from build123d import *

# Parameters (mm, degrees)
F1_R     = 2
F1_W     = 3
F1_H     = 3
F6_DEPTH = 1
F7_DEPTH = 1.6
F5_W     = 3
F5_H     = 3
F8_DEPTH = 1


with BuildPart() as f6:
    # F1 (on Top) → F6 (new body, through all)
    with BuildSketch(Plane.XY):
        with BuildLine():
            ThreePointArc((-30.5, -38), (-27.318019, -36.681981), (-26, -33.5))
            ThreePointArc((-26, -33.5), (-29.882129, -29.04262), (-34.830327, -32.275961))
            ThreePointArc((-34.830327, -32.275961), (-34.088744, -36.214943), (-30.5, -38))
        make_face()
        with Locations((-30.5, -33.5)):
            Circle(F1_R, mode=Mode.SUBTRACT)
        with BuildLine():
            ThreePointArc((-34.830327, -32.275961), (-29.882129, -29.04262), (-26, -33.5))
            ThreePointArc((-26, -33.5), (-27.318019, -36.681981), (-30.5, -38))
            Line((-30.5, -38), (56, -38))
            ThreePointArc((56, -38), (51.55486, -32.79948), (57.383959, -29.218101))
            Line((57.383959, -29.218101), (41.486443, -24.079841))
            Line((41.486443, -24.079841), (-32.513557, -24.079841))
            Line((-32.513557, -24.079841), (-34.830327, -32.275961))
        make_face()
        Polygon((-32.513557, 27.920159), (-32.513557, -24.079841), (41.486443, -24.079841), (41.486443, 27.920159), (38.486443, 27.920159), (38.486443, -21.079841), (-29.513557, -21.079841), (-29.513557, 27.920159), align=None)
        with BuildLine():
            ThreePointArc((57.383959, -29.218101), (51.55486, -32.79948), (56, -38))
            ThreePointArc((56, -38), (59.181981, -36.681981), (60.5, -33.5))
            ThreePointArc((60.5, -33.5), (59.638531, -30.852153), (57.383959, -29.218101))
        make_face()
        with Locations((56, -33.5)):
            Circle(F1_R, mode=Mode.SUBTRACT)
        with Locations((-31.013557, 29.420159)):
            Rectangle(F1_W, F1_H)
        with Locations((39.986443, 29.420159)):
            Rectangle(F1_W, F1_H)
    extrude(amount=F6_DEPTH)

    # F3 (on offset) → F7 (join, through all)
    with BuildSketch(Plane.XY.offset(1)):
        Polygon((-31.013557, 27.920159), (-32.513557, 27.920159), (-32.513557, -24.079841), (41.486443, -24.079841), (41.486443, 27.920159), (39.986443, 27.920159), (39.986443, -22.579841), (-31.013557, -22.579841), align=None)
        Polygon((-32.513557, 30.920159), (-32.513557, 27.920159), (-31.013557, 27.920159), (-31.013557, 28.920159), (-29.513557, 28.920159), (-29.513557, 30.920159), align=None)
        Polygon((39.986443, 27.920159), (41.486443, 27.920159), (41.486443, 30.920159), (38.486443, 30.920159), (38.486443, 28.920159), (39.986443, 28.920159), align=None)
    extrude(amount=F7_DEPTH)

    # F5 (on offset) → F8 (join)
    with BuildSketch(Plane.XY.offset(2.6)):
        Polygon((-29.513557, 27.920159), (-32.513557, 27.920159), (-32.513557, -24.079841), (41.486443, -24.079841), (41.486443, 27.920159), (38.486443, 27.920159), (38.486443, -21.079841), (-29.513557, -21.079841), align=None)
        with Locations((-31.013557, 29.420159)):
            Rectangle(F5_W, F5_H)
        with Locations((39.986443, 29.420159)):
            Rectangle(F5_W, F5_H)
    extrude(amount=F8_DEPTH)


solid = f6.part
The listing builds one solid part. Answer for the finished solid, in the listing's coordinates (mm). A direction names the side the tool comes from. Give positions to 0.01 mm unless a question says otherwise; leave off trailing zeros. Loops run counter-clockwise (first coordinate to the right, second up) from the corner with the lowest first, then second, coordinate; pieces in that order, holes last. Notation, with made-up numbers: (-8, 42.25) - (42, 42.25) arc R19 cw to (42, 54.25) - close; hole circle Ø3 at (-35, 84.25). An arc over 180 degrees is marked (long way). Answer as a JSON object with one key per item and string values.
1. A cutting plane is placed at D-D (x = 47.5). Write down the section's boundary in (y, z), then the cut area to 3 significant figures.
Determined:
{"outline": "(-38, 0) - (-26.02, 0) - (-26.02, 1) - (-38, 1) - close", "area": "12.0 mm²"}
2. A cutting plane is placed at A-A (y = 11.5). Write down the section's boundary in (x, z), then the cut area to 3 significant figures.
Determined:
{"outline": "(-32.51, 0) - (-29.51, 0) - (-29.51, 1) - (-31.01, 1) - (-31.01, 2.6) - (-29.51, 2.6) - (-29.51, 3.6) - (-32.51, 3.6) - close; (38.49, 0) - (41.49, 0) - (41.49, 3.6) - (38.49, 3.6) - (38.49, 2.6) - (39.99, 2.6) - (39.99, 1) - (38.49, 1) - close", "area": "16.8 mm²"}
3. A cutting plane is placed at B-B (x = 20). Write down the section's boundary in (y, z), then the cut area to 3 significant figures.
Determined:
{"outline": "(-38, 0) - (-21.08, 0) - (-21.08, 1) - (-22.58, 1) - (-22.58, 2.6) - (-21.08, 2.6) - (-21.08, 3.6) - (-24.08, 3.6) - (-24.08, 1) - (-38, 1) - close", "area": "22.3 mm²"}
4. Find the intervals of material crossed by L1, parallel to X at y = 23, z = 1.1; L2, parallel to Y at x = -30.5, z = 0.85; L3, parallel to Y at x = -26, z = 1.3, in increasing order. Write a range as [from, to].
Determined:
{"L1": "[-32.51, -31.01], [39.99, 41.49]", "L2": "[-38, -35.5], [-31.5, 30.92]", "L3": "[-24.08, -22.58]"}
5. For faces 1 (the flat face through (-32.514, 4, 2)), 2 (the flat face through (38.486, 5.3, 0.6)), 3 (the flat face through (4, -22, 1)), determine the directions among +Z, -Z, +X, -X, +Y, -Y from which every point of the face is accessible in a straight line to the end or side of a thin tool.
Determined:
{"face 1": "+Z, -Z, -X, +Y", "face 2": "+Z, -Z, +Y", "face 3": "none"}
6. A cutting plane is placed at C-C (y = -27). Write down the section's boundary in (x, z).
Determined:
{"outline": "(-33.34, 0) - (50.52, 0) - (50.52, 1) - (-33.34, 1) - close"}
7. For a pull along X with two mould halves and no side action, classify faces 4 (the flat face through (4, -24.08, 2)), 5 (the flat face through (-33.656, -28.121, 0.493)), 6 (the flat face through (49.546, -26.685, 0.493)), 7 (the flat face through (4, -22, 2.6)) as pulls with the +X half, pulls with the -X half, needs draft (parallel to the pull), parting line crosses it, or undercut.
Determined:
{"face 4": "needs draft", "face 5": "pulls with the -X half", "face 6": "pulls with the +X half", "face 7": "undercut"}
8. Flat-ended cylindrical pins translate along their axes: pin 1 Ø2 at (x, z) = (10, 1.5) entering from -Y; pin 2 Ø1.8 at (y, z) = (3, 1.5) entering from +X; pin 3 Ø2 at (x, z) = (5.5, 3) entering from -Y; pin 4 Ø0.5 at (x, z) = (4, 0.5) entering from +Y. Find the tip coordinate at first contact, or state that the pin passes through.
Determined:
{"pin 1": "y = -38", "pin 2": "x = 41.49", "pin 3": "y = -24.08", "pin 4": "y = -21.08"}
